from build123d import *

# Parameters (mm, degrees)
F0_R     = 1.125
F1_DEPTH = 40
F0_R_2   = 2
F0_R_3   = 2.5
F2_DEPTH = 3
F0_R_4   = 1.1
F3_DEPTH = 10
F4_DEPTH = 3
F5_R     = 5
F6_DEPTH = 4
F7_DEPTH = 25


with BuildPart() as f1:
    # F0 (on Top) → F1 (new body)
    with BuildSketch(Plane.XY):
        with BuildLine():
            Line((-2, 120), (-75, 120))
            ThreePointArc((-75, 120), (-76.414214, 119.414214), (-77, 118))
            Line((-77, 118), (-77, 2))
            ThreePointArc((-77, 2), (-76.414214, 0.585786), (-75, 0))
            Line((-75, 0), (-2, 0))
            ThreePointArc((-2, 0), (-0.585786, 0.585786), (0, 2))
            Line((0, 2), (0, 118))
            ThreePointArc((0, 118), (-0.585786, 119.414214), (-2, 120))
        make_face()
        with Locations((-74.914214, 2.085786)):
            Circle(F0_R, mode=Mode.SUBTRACT)
        with Locations((-2.085786, 2.085786)):
            Circle(F0_R, mode=Mode.SUBTRACT)
        with BuildLine():
            Line((-72, 117), (-38.5, 117))
            Line((-38.5, 117), (-5, 117))
            ThreePointArc((-5, 117), (-3.585786, 116.414214), (-3, 115))
            Line((-3, 115), (-3, 60))
            Line((-3, 60), (-3, 5))
            ThreePointArc((-3, 5), (-3.585786, 3.585786), (-5, 3))
            Line((-5, 3), (-38.5, 3))
            Line((-38.5, 3), (-72, 3))
            ThreePointArc((-72, 3), (-73.414214, 3.585786), (-74, 5))
            Line((-74, 5), (-74, 60))
            Line((-74, 60), (-74, 115))
            ThreePointArc((-74, 115), (-73.414214, 116.414214), (-72, 117))
        make_face(mode=Mode.SUBTRACT)
        with Locations((-74.914214, 117.914214)):
            Circle(F0_R, mode=Mode.SUBTRACT)
        with Locations((-2.085786, 117.914214)):
            Circle(F0_R, mode=Mode.SUBTRACT)
    extrude(amount=F1_DEPTH)

    # F0 (on Top) → F2 (join)
    with BuildSketch(Plane.XY):
        with BuildLine():
            Line((-5, 117), (-38.5, 117))
            Line((-38.5, 117), (-72, 117))
            ThreePointArc((-72, 117), (-73.414214, 116.414214), (-74, 115))
            Line((-74, 115), (-74, 60))
            Line((-74, 60), (-74, 5))
            ThreePointArc((-74, 5), (-73.414214, 3.585786), (-72, 3))
            Line((-72, 3), (-38.5, 3))
            Line((-38.5, 3), (-5, 3))
            ThreePointArc((-5, 3), (-3.585786, 3.585786), (-3, 5))
            Line((-3, 5), (-3, 60))
            Line((-3, 60), (-3, 115))
            ThreePointArc((-3, 115), (-3.585786, 116.414214), (-5, 117))
        make_face()
        with Locations((-70, 7)):
            Circle(F0_R_2, mode=Mode.SUBTRACT)
        with Locations((-62.4, 6)):
            Circle(F0_R_3, mode=Mode.SUBTRACT)
        with Locations((-67.4, 57.5)):
            Circle(F0_R_3, mode=Mode.SUBTRACT)
        with Locations((-33.9, 6)):
            Circle(F0_R_3, mode=Mode.SUBTRACT)
        with Locations((-7, 7)):
            Circle(F0_R_2, mode=Mode.SUBTRACT)
        with Locations((-19.4, 57.4)):
            Circle(F0_R_3, mode=Mode.SUBTRACT)
        with Locations((-70, 113)):
            Circle(F0_R_2, mode=Mode.SUBTRACT)
        with Locations((-7, 113)):
            Circle(F0_R_2, mode=Mode.SUBTRACT)
    extrude(amount=F2_DEPTH)

    # F0 (on Top) → F3 (join)
    with BuildSketch(Plane.XY):
        with Locations((-67.4, 57.5)):
            Circle(F0_R_3)
        with Locations((-67.4, 57.5)):
            Circle(F0_R_4, mode=Mode.SUBTRACT)
        with Locations((-19.4, 57.4)):
            Circle(F0_R_3)
        with Locations((-19.4, 57.4)):
            Circle(F0_R_4, mode=Mode.SUBTRACT)
        with Locations((-33.9, 6)):
            Circle(F0_R_3)
        with Locations((-33.9, 6)):
            Circle(F0_R_4, mode=Mode.SUBTRACT)
        with Locations((-62.4, 6)):
            Circle(F0_R_3)
        with Locations((-62.4, 6)):
            Circle(F0_R_4, mode=Mode.SUBTRACT)
    extrude(amount=F3_DEPTH)

    # F0 (on Top) → F4 (join)
    with BuildSketch(Plane.XY):
        with Locations((-67.4, 57.5)):
            Circle(F0_R_4)
        with Locations((-19.4, 57.4)):
            Circle(F0_R_4)
        with Locations((-33.9, 6)):
            Circle(F0_R_4)
        with Locations((-62.4, 6)):
            Circle(F0_R_4)
    extrude(amount=F4_DEPTH)

    # F5 (on Front) → F6 (cut)
    with BuildSketch(Plane.XZ):
        with Locations((-20.117393, 20)):
            Circle(F5_R)
    extrude(amount=-F6_DEPTH, mode=Mode.SUBTRACT)

    # F0 (on Top) → F7 (join)
    with BuildSketch(Plane.XY):
        with Locations((-74.914214, 117.914214)):
            Circle(F0_R)
        with Locations((-2.085786, 117.914214)):
            Circle(F0_R)
        with Locations((-2.085786, 2.085786)):
            Circle(F0_R)
        with Locations((-74.914214, 2.085786)):
            Circle(F0_R)
    extrude(amount=F7_DEPTH)


solid = f1.part
The listing builds one solid part. Answer for the finished solid, in the listing's coordinates (mm). A direction names the side the tool comes from. Coordinates: 2 decimals unless noted, no trailing zeros. Order: outer loops, then holes, each group sorted by start corner. A loop starts at its lowest first (then second) coordinate and runs counter-clockwise, first axis right, second up. Notation, with made-up numbers: M -11.5,73 L 21.5,73 A20 cw 21.5,77 Z; hole C 76,36.5 d3. An arc over 180 degrees is marked long. Use CSV: the item, a comma, the result in double quotes.
Q1. A tool of negligible diameter and unlimited length cuts with its end or side. For faces 4 (the flat face through (-39, 61, 0)), 5 (the flat face through (-74, 59, 21)), from which of +Z, -Z, +X, -X, +Y, -Y can it reach the whole face along a straight path? Write none if from no direction.
Here are the results:
face 4,"-Z, +X, -X, +Y, -Y"
face 5,"+Z"
Q2. Section D-D (x = -7) is taken. Determine the outline of the cut face in (y, z).
Here are the results:
outline,"M 0,0 L 5,0 L 5,3 L 3,3 L 3,40 L 0,40 Z; M 9,0 L 111,0 L 111,3 L 9,3 Z; M 115,0 L 120,0 L 120,40 L 117,40 L 117,3 L 115,3 Z"
Q3. Section B-B (y = 113) is taken. Determine the outline of the cut face in (x, z), then the cut area to 3 significant figures.
Here are the results:
outline,"M -77,0 L -72,0 L -72,3 L -74,3 L -74,40 L -77,40 Z; M -68,0 L -9,0 L -9,3 L -68,3 Z; M -5,0 L 0,0 L 0,40 L -3,40 L -3,3 L -5,3 Z"
area,"429 mm2"
Q4. Determine the mould class of faces 1 (the cylindrical face through (-68.925, 114.686, 1.479)), 2 (the cylindrical face through (-21.2, 1.48, 15.12)), 3 (the flat face through (-67, 56, 10)) for opening direction Z: pulls with the +Z half, pulls with the -Z half, needs draft (parallel to the pull), parting line crosses it, or undercut.
Here are the results:
face 1,"needs draft"
face 2,"undercut"
face 3,"pulls with the +Z half"
Q5. Straight lines are drawn through the part: L1, parallel to X at y = 9.5, z = 35.5; L2, parallel to Y at x = -39.5, z = 8; L3, parallel to Y at x = -70, z = 1.25. For each, find the intervals that lie inside material, in ascending order.
Here are the results:
L1,"-77 to -74, -3 to 0"
L2,"0 to 3, 117 to 120"
L3,"0 to 5, 9 to 111, 115 to 120"
Q6. Section A-A (z = 4.5) is taken. Give the number of separate pieces and of enclosed holes in the cut face, then the cut area to 3 significant figures.
Here are the results:
separate pieces,"5"
enclosed holes,"5"
area,"1,210 mm2"
Q7. Section C-C (x = -48) is taken. Determine the outline of the cut face in (y, z), then the cut area to 3 significant figures.
Here are the results:
outline,"M 0,0 L 120,0 L 120,40 L 117,40 L 117,3 L 3,3 L 3,40 L 0,40 Z"
area,"582 mm2"
Q8. Given pin 1 Ø10 at (x, y) = (-41, 92.5) entering from +Z; pin 2 Ø2.5 at (x, y) = (-70, 7) entering from -Z; pin 3 Ø5.5 at (x, y) = (-19.5, 58) entering from +Z; pin 4 Ø9 at (x, z) = (-20.12, 20) entering from -Y, each flat-ended and moving along its own axis, determine where each tip first touches the part or whether it passes through.
Here are the results:
pin 1,"z = 3"
pin 2,"through"
pin 3,"z = 10"
pin 4,"y = 117"
